Autodesk Inventor part; units mm, degrees
ref_plane "YZ Plane" through (0, 0, 0) normal (1, 0, 0) x (0, 1, 0)
ref_plane "XZ Plane" through (0, 0, 0) normal (0, 1, 0) x (-1, 0, 0)
ref_plane "XY Plane" through (0, 0, 0) normal (0, 0, 1) x (1, 0, 0)
sketch "Sketch1" plane through (0, 0, 0) normal (0, 0, 1) x (1, 0, 0)
  circle A0 centre (0, 0) radius 142.5
  dimension "d22" = 285
extrude "Plate1" add sketch "Sketch1" along normal blind 3
sketch "Sketch5" plane through (0, 0, 3) normal (0, 0, 1) x (1, 0, 0)
  circle A0 centre (0, 0) radius 142.5
  circle A1 centre (0, 120.5) radius 9
  circle A2 centre (0, 0) radius 120.5 construction
  dimension "d23" = 18
  dimension "d30" = 22
extrude "Cut1" cut sketch "Sketch5" against normal blind 3 contours A1
pattern_circular "Circular Pattern1" count 8 over 360 about axis through (0, 0, 0) along (0, 0, 1) of "Cut1"
equation "\"d25\" = Thickness"
equation "\"d2\" = Thickness"
equation "\"BendReliefWidth\" = Thickness"
equation "\"BendReliefDepth\" = 0.5 * Thickness"
equation "\"CornerReliefSize\" = 4 * Thickness"
equation "\"MinimumRemnant\" = 2 * Thickness"
equation "\"TransitionRadius\" = BendRadius"
equation "\"JacobiRadiusSize\" = BendRadius"
equation "\"GapSize\" = Thickness"
properties part number "MSC 922 plug 150" material "Stainless Steel"
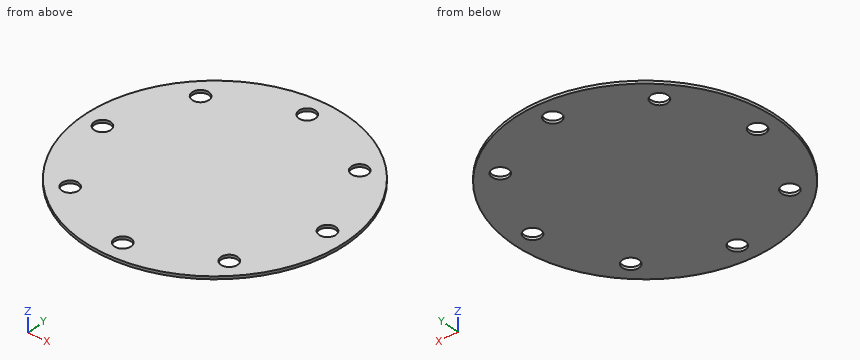
Could you check a few things on this model? Use its own coordinates, in mm. Round coordinates to 2 decimals unless told otherwise and drop trailing zeros. Order: outer loops, then holes, each group sorted by start corner. A loop starts at its lowest first (then second) coordinate and runs counter-clockwise, first axis right, second up. Notation, with made-up numbers: M 75.25,18.5 L 107.25,18.5 A22 ccw 107.25,55.5 Z; hole C 88,74 d8. An arc over 180 degrees is marked long. One line per item, written item: value.
(1) Imagine slicing it at C-C (z = 1.2). Count the separate pieces of the cut face and the enclosed holes in it, and give its area (3 significant figures).
Ans:
separate pieces: 1
enclosed holes: 8
area: 61,800 mm^2
(2) I'm going to push flat-ended pins straight in: P1, Ø23.5, axis at x = 85.21, y = 85.21, coming from the -Z side; P2, Ø16, axis at x = -85.21, y = -85.21, coming from the +Z side; P3, Ø1, axis at x = 61.5, z = 1.5, coming from the -Y side. Where does each tip first touch, or does it pass through?
Ans:
P1: stops at z = 0
P2: passes through
P3: stops at y = -128.78
(3) I need wall thicknesses on line 1 along Y through (x, z) = (79, 0.4); line 2 along Y through (x, z) = (-59.5, 2.55); line 3 along Y through (x, z) = (83.5, 1.4). Which ranges of each line are inside material? Lowest first, please. Write a range as from..to.
Ans:
line 1: y = -118.6..-91.72, -78.69..78.69, 91.72..118.6
line 2: y = -129.48..129.48
line 3: y = -115.47..-94.04, -76.37..76.37, 94.04..115.47
(4) Imagine slicing it at D-D (y = -120.5). Write out the boundary of the cut face in (x, z), and give its area (3 significant figures).
Ans:
outline: M -76.07,0 L -9,0 L -9,3 L -76.07,3 Z; M 9,0 L 76.07,0 L 76.07,3 L 9,3 Z
area: 402 mm^2
(5) Imagine slicing it at A-A (y = 0). Write out the boundary of the cut face in (x, z), and give its area (3 significant figures).
Ans:
outline: M -142.5,0 L -129.5,0 L -129.5,3 L -142.5,3 Z; M -111.5,0 L 111.5,0 L 111.5,3 L -111.5,3 Z; M 129.5,0 L 142.5,0 L 142.5,3 L 129.5,3 Z
area: 747 mm^2
